The model under review builds one solid part; all positions refer to its coordinate system, in mm. A direction names the side the tool comes from. Round coordinates to 2 decimals unless told otherwise and drop trailing zeros. Write each loop counter-clockwise with the first axis right and the second up, starting at its lowest first coordinate (ties: lowest second). Pieces come first, ordered by that corner, then holes. Notation, with made-up numbers: (12.25, 17.5) - (61.25, 17.5) arc R22 cw to (61.25, 42.5) - close; hole circle Ø2 at (-9.75, 85). An arc over 180 degrees is marked (long way). Write each question's results on one line, items separated by ' | '.
Autodesk Inventor part; units mm, degrees
ref_plane "YZ Plane" through (0, 0, 0) normal (1, 0, 0) x (0, 1, 0)
ref_plane "XZ Plane" through (0, 0, 0) normal (0, 1, 0) x (-1, 0, 0)
ref_plane "XY Plane" through (0, 0, 0) normal (0, 0, 1) x (1, 0, 0)
sketch "Sketch1" plane through (0, 0, 0) normal (0, 1, 0) x (-1, 0, 0)
  arc A0 (8.5, 13.7081) -> (11.5, 13.7081) centre (10, 10) ccw
  line L0 (8.5, 20) -> (8.5, 13.7081)
  line L1 (11.5, 20) -> (11.5, 13.7081)
  line L2 (10, 20) -> (10, 18.7339)
  line L3 (20, 20) -> (10, 20)
  line L4 (8.5, 20) -> (0, 20)
  line L5 (0, 20) -> (0, 0)
  line L6 (0, 0) -> (20, 0)
  line L7 (20, 0) -> (20, 20)
  arc A1 (68.5, 13.7081) -> (71.5, 13.7081) centre (70, 10) ccw
  line L8 (68.5, 20) -> (68.5, 13.7081)
  line L9 (71.5, 20) -> (71.5, 13.7081)
  line L10 (70, 20) -> (70, 18.3732)
  line L11 (80, 20) -> (70, 20)
  line L12 (68.5, 20) -> (60.9559, 20)
  line L13 (60.9559, 20) -> (60.9559, 0)
  line L14 (60.9559, 0) -> (80, 0)
  line L15 (80, 0) -> (80, 20)
  line L16 (60.9559, 0) -> (20, 0)
  line L17 (20, 0) -> (20, 20)
  line L18 (20, 20) -> (60.9559, 20)
  line L19 (60.9559, 20) -> (60.9559, 0)
  dimension "d2" = 8
  dimension "d7" = 1.5
  dimension "d8" = 1.5
  dimension "d16" = 10
  dimension "d17" = 8
  dimension "d18" = 1.5
  dimension "d19" = 1.5
  dimension "d20" = 10
  dimension "d22" = 80
  dimension "d23" = 10
  dimension "d24" = 0
  dimension "d25" = 60
  dimension "d26" = 20
  dimension "d27" = 20
  dimension "d28" = 20
  dimension "d29" = 20
  dimension "d30" = 10
  dimension "d31" = 10
  dimension "d32" = 20
extrude "Extrusion1" add sketch "Sketch1" along normal blind 36
sketch "Sketch5" plane through (-80, 0, 0) normal (-1, 0, 0) x (0, 0, 1)
  line L0 (20, 0) -> (20, 36)
  line L1 (20, 36) -> (-15, 36)
  line L2 (-15, 6) -> (20, 6)
  line L3 (20, 6) -> (20, 36)
  line L4 (-15, 36) -> (-15, 29.1398)
  line L5 (-15, 12.9843) -> (-15, 6)
  line L6 (0, 0) -> (0, 36)
  line L7 (0, 0) -> (0, 36)
  line L8 (0, 6) -> (0, 36)
  arc A0 (-15, 12.9843) -> (-15, 29.1398) centre (-10, 21.062) ccw
  dimension "d40" = 30
  dimension "d41" = 35
  dimension "d45" = 20
  dimension "d85" = 19
  dimension "d86" = 5
  dimension "d87" = 15
extrude "Extrusion5" add sketch "Sketch5" against normal blind 80 contours L2 L5 A0 L4 L1 L6
sketch "Sketch13" plane through (0, 36, 0) normal (0, 1, 0) x (1, 0, 0)
  line L0 (-80, -20) -> (-80, 15)
  line L1 (-80, -20) -> (-71.5, -20)
  line L2 (-71.5, -20) -> (-71.5, -13.7081)
  arc A0 (-68.5, -13.7081) -> (-71.5, -13.7081) centre (-70, -10) ccw
  line L3 (-68.5, -13.7081) -> (-68.5, -20)
  line L4 (-68.5, -20) -> (-11.5, -20)
  line L5 (-11.5, -20) -> (-11.5, -13.7081)
  arc A1 (-8.5, -13.7081) -> (-11.5, -13.7081) centre (-10, -10) ccw
  line L6 (-8.5, -13.7081) -> (-8.5, -20)
  line L7 (-8.5, -20) -> (0, -20)
  line L8 (0, -20) -> (0, 15)
  line L9 (-80, 15) -> (0, 15)
  point P0 (0, 0)
extrude "Extrusion11" cut sketch "Sketch13" against normal blind 1
sketch "Sketch16" plane through (-80, 6, -15) normal (0, 0, -1) x (-1, 0, 0)
  line L0 (-80, -6) -> (0, -6)
  line L1 (0, 6.9843) -> (-80, 6.9843)
  line L2 (-80, -6) -> (0, -6)
  line L3 (0, -6) -> (0, 6.9843)
  line L4 (0, 6.9843) -> (-80, 6.9843)
  line L5 (-80, 6.9843) -> (-80, -6)
  line L6 (0, -6) -> (0, 29)
  line L7 (0, 23.1398) -> (-80, 23.1398)
  line L8 (0, 29) -> (-80, 29)
  line L9 (-80, 29) -> (-80, 23.1398)
  line L10 (-80, 23.1398) -> (0, 23.1398)
  line L11 (0, 23.1398) -> (0, 29)
extrude "Extrusion13" add sketch "Sketch16" along normal blind 6
sketch "Sketch17" plane through (0, 0, 0) normal (0, 0, -1) x (-1, 0, 0)
  line L0 (80, 6) -> (0, 6)
  line L1 (0, 0) -> (80, 0)
  line L2 (80, 6) -> (0, 6)
  line L3 (80, 6) -> (80, 0)
  line L4 (0, 6) -> (0, 0)
extrude "Extrusion14" add sketch "Sketch17" along normal blind 20
sketch "Sketch18" plane through (-68.5, 0, 20) normal (0, 0, 1) x (1, 0, 0)
  line L0 (13.5, 0) -> (43.5, 0)
  line L1 (43.5, 0) -> (43.5, 15)
  line L2 (43.5, 15) -> (13.5, 15)
  line L3 (13.5, 15) -> (13.5, 0)
  line L4 (-11.5, 0) -> (-11.5, 35)
  line L5 (0, 0) -> (57, 0)
  point P0 (68.5, 0)
  dimension "d107" = 30
  dimension "d108" = 25
  dimension "d109" = 15
  dimension "d110" = 0
extrude "Extrusion15" cut sketch "Sketch18" against normal blind 37
sketch "Sketch19" plane through (0, 0, 0) normal (0, -1, 0) x (1, 0, 0)
  line L0 (-80, -21) -> (0, -21)
  line L1 (-30, -21) -> (-23, -21)
  line L2 (-23, -21) -> (-23, -44)
  line L3 (-23, -44) -> (-30, -44)
  line L4 (-30, -44) -> (-30, -21)
  line L5 (-30, -44) -> (-50, -44)
  line L6 (-50, -44) -> (-50, -39)
  line L7 (-50, -39) -> (-30, -39)
  line L8 (-30, -39) -> (-30, -44)
  line L9 (-50, -44) -> (-57, -44)
  line L10 (-57, -44) -> (-57, -21)
  line L11 (-57, -21) -> (-50, -21)
  line L12 (-50, -21) -> (-50, -44)
  line L13 (0, -21) -> (0, 20)
  point P0 (0, 0)
  dimension "d113" = 7
  dimension "d114" = 7
  dimension "d115" = 5
  dimension "d116" = 18
  dimension "d117" = 20
  dimension "d118" = 23
extrude "Extrusion16" add sketch "Sketch19" against normal blind 15.5 contours L0 L12 L6 L9 L10 | L0 L2 L3 L4 | L7 L4 L5 L6
sketch "Sketch20" plane through (-23, 0, -44) normal (0, 0, -1) x (-1, 0, 0)
  circle A0 centre (17, 7.5) radius 1.75
  line L0 (34, 0) -> (0, 0)
  line L1 (-23, 12.9843) -> (-23, 0)
  dimension "d121" = 3.5
  dimension "d122" = 7.5
  dimension "d123" = 40
extrude "Extrusion17" cut sketch "Sketch20" against normal blind 80
sketch "Sketch21" plane through (0, 0, 0) normal (0, -1, 0) x (1, 0, 0)
  line L0 (0, -0.5) -> (-80, -0.5)
  line L1 (0, -21) -> (-23, -21)
  line L2 (0, -21) -> (0, 20)
  line L3 (0, 20) -> (-8.5, 20)
  line L4 (-8.5, 20) -> (-8.5, 13.7081)
  arc A0 (-11.5, 13.7081) -> (-8.5, 13.7081) centre (-10, 10) ccw
  line L5 (-11.5, 13.7081) -> (-11.5, 20)
  line L6 (-25, 20) -> (-11.5, 20)
  line L7 (-25, 20) -> (-25, -17)
  line L8 (-25, -17) -> (-55, -17)
  line L9 (-55, -17) -> (-55, 20)
  line L10 (-68.5, 20) -> (-55, 20)
  line L11 (-68.5, 13.7081) -> (-68.5, 20)
  arc A1 (-71.5, 13.7081) -> (-68.5, 13.7081) centre (-70, 10) ccw
  line L12 (-71.5, 20) -> (-71.5, 13.7081)
  line L13 (-80, 20) -> (-71.5, 20)
  line L14 (-80, 20) -> (-80, -21)
  line L15 (-57, -21) -> (-80, -21)
  line L16 (-57, -21) -> (-57, -44)
  line L17 (-57, -44) -> (-23, -44)
  line L18 (-23, -44) -> (-23, -21)
  line L19 (-30, -21) -> (-30, -39)
  line L20 (-30, -39) -> (-50, -39)
  line L21 (-50, -39) -> (-50, -21)
  line L22 (-30, -21) -> (-50, -21)
  point P0 (0, 0)
extrude "Extrusion18" cut sketch "Sketch21" against normal blind 2.5 contours L2 L1 L18 L17 L16 L15 L14 L0 L9 L8 L7 | L0 L7 L6 L5 A0 L4 L3 L2 | L0 L14 L13 L12 A1 L11 L10 L9 | L19 L20 L21 L22
sketch "Sketch22" plane through (-68.5, 35, 20) normal (0, 0, 1) x (1, 0, 0)
  line L0 (0, -32.5) -> (13.5, -32.5)
  line L1 (13.5, -32.5) -> (13.5, -20)
  line L2 (13.5, -20) -> (43.5, -20)
  line L3 (43.5, -20) -> (43.5, -32.5)
  line L4 (43.5, -32.5) -> (57, -32.5)
  line L5 (57, -32.5) -> (57, 0)
  line L6 (57, 0) -> (0, 0)
  line L7 (0, -32.5) -> (0, 0)
  line L8 (60, -32.5) -> (68.5, -32.5)
  line L9 (68.5, -32.5) -> (68.5, 0)
  line L10 (68.5, 0) -> (60, 0)
  line L11 (60, -32.5) -> (60, 0)
  line L12 (-11.5, -32.5) -> (-3, -32.5)
  line L13 (-3, -32.5) -> (-3, 0)
  line L14 (-3, 0) -> (-11.5, 0)
  line L15 (-11.5, -32.5) -> (-11.5, 0)
  point P0 (68.5, -35)
extrude "Extrusion19" add sketch "Sketch22" along normal blind 15
sketch "Sketch23" plane through (-68.5, 35, 35) normal (0, 0, 1) x (1, 0, 0)
  line L0 (-11.5, 0) -> (68.5, 0)
  line L1 (48.5, 0) -> (8.5, 0)
  line L2 (8.5, 0) -> (8.5, -32.5)
  line L3 (8.5, -32.5) -> (48.5, -32.5)
  line L4 (48.5, -32.5) -> (48.5, 0)
  line L5 (68.5, -32.5) -> (68.5, 0)
  line L6 (-11.5, 0) -> (-11.5, -32.5)
  point P0 (57, 0)
  point P1 (8.5, 0)
  dimension "d130" = 20
  dimension "d131" = 20
extrude "Extrusion20" cut sketch "Sketch23" against normal blind 20
sketch "Sketch24" plane through (0, 15.5, 0) normal (0, 1, 0) x (1, 0, 0)
  line L0 (-23, 21) -> (-23, 44)
  line L1 (-23, 44) -> (-57, 44)
  line L2 (-57, 44) -> (-57, 21)
  line L3 (-57, 21) -> (-50, 21)
  line L4 (-50, 21) -> (-50, 39)
  line L5 (-50, 39) -> (-30, 39)
  line L6 (-30, 39) -> (-30, 21)
  line L7 (-30, 21) -> (-23, 21)
  point P0 (0, 0)
extrude "Extrusion21" cut sketch "Sketch24" against normal blind 2.5
equation "\"d2\" = RodDiameter"
equation "\"d17\" = d2"
equation "\"d85\" = XLinearBearingOD"
equation "\"RodDiameter\" = 8"
equation "\"VerticalBearingOD\" = 16"
equation "\"PrintingClearance\" = 0.2"
equation "\"d21\" = 8"
equation "\"TubeID\" = 18"
equation "\"XLinearBearingOD\" = 19"
properties part number "GantryHolder" material "PET Plastic"
Q1. Insertion check: P1, Ø7, axis at x = -10, z = 10, coming from the +Y side; P2, Ø5, axis at y = 6, z = -37, coming from the -X side; P3, Ø6, axis at x = -54, y = 31, coming from the +Z side; P4, Ø18.5, axis at x = -33, z = -35, coming from the +Y side. Each pin has a flat end and moves straight along its axis. Give the tip position at first contact, or say it passes through.
Evaluation:
P1: passes through | P2: stops at x = -57 | P3: stops at z = 15 | P4: stops at y = 13
Q2. Tool access review of faces 1 (the flat face through (-8.5, 19, 25)), 2 (the flat face through (-41, 29.14, -18)), 3 (the flat face through (-30, 8, -30)), 4 (the flat face through (-40, 10, -17)): name each direction out of +Z, -Z, +X, -X, +Y, -Y from which nothing blocks a thin tool from reaching the whole face with its end or side.
Evaluation:
face 1: +Z, +Y, -Y | face 2: -Z, +X, -X | face 3: +Y, -Y | face 4: +Z, -Y
Q3. For probe 1 along X at (y, z) = (21, 19.5); probe 2 along Y at (x, z) = (-40, -41); probe 3 along Z at (x, y) = (-31.5, 12), list the stretches that pass through material, from the lowest coordinate up.
Evaluation:
probe 1: x = -80 to -71.5, -68.5 to -60, -20 to -11.5, -8.5 to 0 | probe 2: y = 2.5 to 5.75, 9.25 to 13 | probe 3: z = -44 to -39, -21 to -17
Q4. We need section B-B (x = -40). State the section outline as (y, z) points.
Evaluation:
outline: (2.5, -44) - (5.75, -44) - (5.75, -39) - (2.5, -39) - close; (2.5, -21) - (5.75, -21) - (5.75, -17) - (2.5, -17) - close; (9.25, -44) - (13, -44) - (13, -39) - (9.25, -39) - close; (9.25, -21) - (12.98, -21) - (12.98, -17) - (9.25, -17) - close; (15, -2.69) arc R9.5 cw to (29.14, -15) - (29.14, -21) - (35, -21) - (35, 15) - (15, 15) - close
Q5. The part is to be moulded in two halves that separate along X. For faces 5 (the flat face through (-11.5, 19, 25)), 6 (the flat face through (-57, 8, -33)), 7 (the flat face through (-64, 19, 35)), say which applies: released by +X, released by -X, zero draft, split by the parting line, or undercut.
Evaluation:
face 5: undercut | face 6: released by -X | face 7: zero draft
Q6. We need section A-A (z = 10). State the section outline as (x, y) points, plus the area to 4 significant figures.
Evaluation:
outline: (-80, 2.5) - (-74, 2.5) - (-74, 35) - (-80, 35) - close; (-66, 2.5) - (-55, 2.5) - (-55, 15) - (-25, 15) - (-25, 2.5) - (-14, 2.5) - (-14, 35) - (-66, 35) - close; (-6, 2.5) - (0, 2.5) - (0, 35) - (-6, 35) - close | area: 1,705 mm^2
Q7. We need section C-C (z = 18). State the section outline as (x, y) points, plus the area to 4 significant figures.
Evaluation:
outline: (-80, 2.5) - (-71.5, 2.5) - (-71.5, 35) - (-80, 35) - close; (-68.5, 2.5) - (-60, 2.5) - (-60, 35) - (-68.5, 35) - close; (-20, 2.5) - (-11.5, 2.5) - (-11.5, 35) - (-20, 35) - close; (-8.5, 2.5) - (0, 2.5) - (0, 35) - (-8.5, 35) - close | area: 1,105 mm^2
Q8. We need section D-D (y = 18.5). State the section outline as (x, z) points.
Evaluation:
outline: (-80, -0.85) - (0, -0.85) - (0, 35) - (-8.5, 35) - (-8.5, 13.71) arc R4 cw (long way) to (-11.5, 13.71) - (-11.5, 35) - (-20, 35) - (-20, 15) - (-60, 15) - (-60, 35) - (-68.5, 35) - (-68.5, 13.71) arc R4 cw (long way) to (-71.5, 13.71) - (-71.5, 35) - (-80, 35) - close
